For this review, take the finished solid that the model builds, in its own axes (mm). Face numbers are marked on the shaded views. A direction names the side the tool comes from. Round coordinates to 2 decimals unless told otherwise and drop trailing zeros. Write each loop counter-clockwise with the first axis right and the second up, starting at its lowest first coordinate (ties: lowest second). Pieces come first, ordered by that corner, then holes.
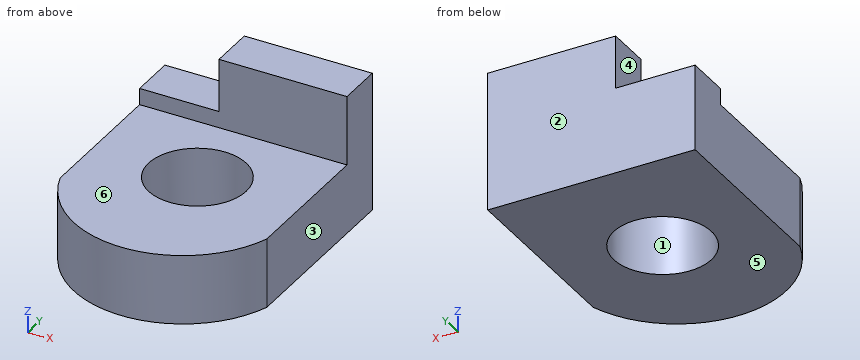
from build123d import *

# Parameters (mm, degrees)
F1_DEPTH = 12.7
F2_W     = 37.782497704
F2_H     = 8.2107339986
F3_DEPTH = 12.7
F4_W     = 14.4625585526
F4_H     = 9.6896222413
F5_DEPTH = 8.2117339986
F6_R     = 8.89
F7_DEPTH = 12.701


with BuildPart() as f1:
    # F0 (on Top) → F1 (new body)
    with BuildSketch(Plane.XY):
        with BuildLine():
            Line((18.891248852, -11.1125009134), (18.891248852, 23.1139999814))
            Line((18.891248852, 23.1139999814), (-18.891248852, 23.1139999814))
            Line((-18.891248852, 23.1139999814), (-18.891248852, -10.8902500942))
            ThreePointArc((-18.891248852, -10.8902500942), (-0.0802847481, -24.6497315476), (18.891248852, -11.1125009134))
        make_face()
    extrude(amount=F1_DEPTH)

    # F2 (on face) → F3 (join)
    with BuildSketch(Plane.XY.offset(12.7)):
        with Locations((0, 19.0086329821)):
            Rectangle(F2_W, F2_H)
    extrude(amount=F3_DEPTH)

    # F4 (on face) → F5 (cut, through all)
    with BuildSketch(Plane.XZ.offset(-14.9032659829)):
        with Locations((-11.6599695757, 20.5551888794)):
            Rectangle(F4_W, F4_H)
    extrude(amount=-F5_DEPTH, mode=Mode.SUBTRACT)

    # F6 (on face) → F7 (cut, through all)
    with BuildSketch(Plane.XY.offset(12.7)):
        Circle(F6_R)
    extrude(amount=-F7_DEPTH, mode=Mode.SUBTRACT)


solid = f1.part
(1) For line 1 along Y through (x, z) = (0, 6.75); line 2 along Z through (x, y) = (10.5, -2); line 3 along Y through (x, z) = (1.5, 14.75), list the stretches that pass through material, from the lowest coordinate up.
Geometry check:
line 1: y = -24.65 to -8.89, 8.89 to 23.11
line 2: z = 0 to 12.7
line 3: y = 14.9 to 23.11
(2) We need section C-C, the plane x = 0. Give the boundary of the cut face in (y, z), and give its area (3 significant figures).
Geometry check:
outline: (-24.65, 0) - (-8.89, 0) - (-8.89, 12.7) - (-24.65, 12.7) - close; (8.89, 0) - (23.11, 0) - (23.11, 25.4) - (14.9, 25.4) - (14.9, 12.7) - (8.89, 12.7) - close
area: 485 mm2
(3) For the marked faces 4, 5 and 6, list the 3-axis set-ups (+Z, -Z, +X, -X, +Y, -Y) from which the entire face can be reached by the end or side of a thin tool; tool diameter is ignored.
Geometry check:
face 4: +Z, -X, +Y, -Y
face 5: -Z, +X, -X, +Y, -Y
face 6: +Z, +X, -X, -Y
(4) For pin 1 Ø2.5 at (x, y) = (-8, 17) entering from +Z; pin 2 Ø6.5 at (x, z) = (-3, 18) entering from -Y; pin 3 Ø4 at (y, z) = (19, 19.5) entering from -X, all flat-tipped, find the tip position at first contact; note any pin that passes through.
Geometry check:
pin 1: stops at z = 15.71
pin 2: stops at y = 14.9
pin 3: stops at x = -4.43
(5) We need section D-D, the plane y = 19.5. Give the boundary of the cut face in (x, z), and give its area (3 significant figures).
Geometry check:
outline: (-18.89, 0) - (18.89, 0) - (18.89, 25.4) - (-4.43, 25.4) - (-4.43, 15.71) - (-18.89, 15.71) - close
area: 820 mm2
(6) We need section A-A, the plane y = -3. Give the boundary of the cut face in (x, z), and give its area (3 significant figures).
Geometry check:
outline: (-18.89, 0) - (-8.37, 0) - (-8.37, 12.7) - (-18.89, 12.7) - close; (8.37, 0) - (18.89, 0) - (18.89, 12.7) - (8.37, 12.7) - close
area: 267 mm2
(7) Mouldability with a two-part tool opening along X and no side actions: class the marked faces 1, 2 and 3 as pulls with the +X half, pulls with the -X half, needs draft (parallel to the pull), parting line crosses it, or undercut.
Geometry check:
face 1: undercut
face 2: needs draft
face 3: pulls with the +X half
(8) We need section B-B, the plane z = 7. Give the boundary of the cut face in (x, y).
Geometry check:
outline: (-18.89, -10.89) arc R19.9 ccw to (18.89, -11.11) - (18.89, 23.11) - (-18.89, 23.11) - close; hole circle Ø17.78 at (0, 0)
